Here's how the part is built. I have some questions about the finished solid (model axes, mm). Face numbers are marked on the shaded views. A direction names the side the tool comes from. Coordinates: 2 decimals unless noted, no trailing zeros. Loops run counter-clockwise (first coordinate to the right, second up) from the corner with the lowest first, then second, coordinate; pieces in that order, holes last. Notation, with made-up numbers: (-19, 16) -> (33, 16) arc R22 ccw to (33, 30) -> close; hole circle Ø10 at (-27.75, -40). An arc over 180 degrees is marked (long way). Answer as a JSON object with one key per item and string values. Group by question number.
1) Which directions (+Z, -Z, +X, -X, +Y, -Y) give clear straight access to the entire face, cutting with the end or side of a thin tool? Please do the marked faces 5, 6, 7, 8 and 9.
2) If we mould it in two halves opening along X, with no side actions, what happens to the marked faces 1, 2, 3 and 4? For each: +X half, -X half, draft (parallel to the pull), parting line (faces both ways), or undercut.
3) I'm going to push flat-ended pins straight in: pin 1 (13.5 mm diameter, centred on x = 23, z = 14.5, fed in from -Y); pin 2 (3.5 mm diameter, centred on x = 9, y = -43, fed in from +Z); pin 3 (10 mm diameter, centred on x = 0.5, y = -2, fed in from -Z). Where does each tip first touch, or does it pass through?
4) I want a section at B-B (x = 7.5). Write out the boundary of the cut face in (y, z).
5) I want a section at D-D (y = -34). Write out the boundary of the cut face in (x, z), then the cut area to 3 significant figures.
6) I need wall thicknesses on probe 1 along Y at (x, z) = (-11.5, 25.5); probe 2 along Z at (x, y) = (9, 3). Which ranges of each line are inside material? Lowest first, please. Write a range as [from, to].
7) I want a section at C-C (z = 6). Write out the boundary of the cut face in (x, y), then the cut area to 3 significant figures.
8) I want a section at A-A (y = 19). Write out the boundary of the cut face in (x, z).
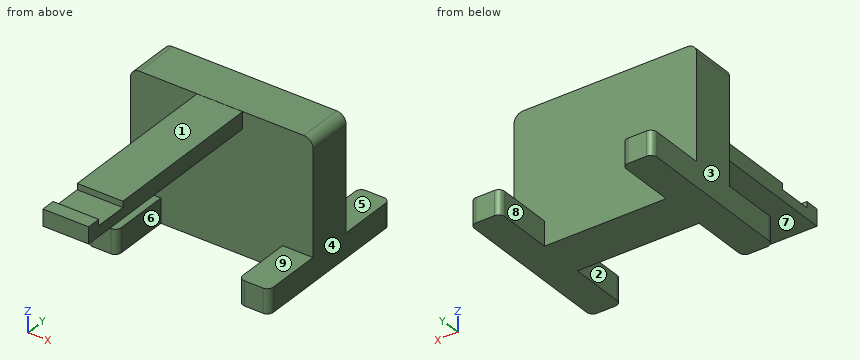
Autodesk Fusion 360 part; units mm, degrees
sketch "Sketch1" plane through (0, 0, 0) normal (0, 0, 1) x (1, 0, 0)
  line L0 (-20, 40) -> (-19.9999, 40)
  line L1 (-19.9999, 10) -> (-20, 10)
  line L2 (-20, 40) -> (40, 40)
  line L3 (40, 40) -> (40, 25)
  line L4 (40, 25) -> (-20, 25)
  line L5 (-20, 25) -> (-20, 40)
  line L6 (20, 40) -> (40, 40)
  dimension "d12" = 60
extrude "Extrude6" add sketch "Sketch1" along normal blind 40
sketch "Sketch5" plane through (0, 25, 0) normal (0, -1, 0) x (1, 0, 0)
  line L0 (-20, 0) -> (40, 0)
  line L1 (40, 0) -> (40, 40)
  line L2 (40, 40) -> (-20, 40)
  line L3 (-20, 40) -> (-20, 0)
  line L4 (1.8726, 40) -> (16.8726, 40)
  line L5 (16.8726, 40) -> (16.8726, 45.446)
  line L6 (16.8726, 45.446) -> (1.8726, 45.446)
  line L7 (1.8726, 45.446) -> (1.8726, 40)
  point P0 (10, 40)
  dimension "d29" = 15
extrude "Extrude7" add sketch "Sketch5" along normal blind 70 contours L2 L4 L5 L6 L7
sketch "Sketch6" plane through (0, 0, 40) normal (0, 0, -1) x (-1, 0, 0)
  line L0 (20, 40) -> (20, 25)
  line L1 (20, 25) -> (-1.8726, 25)
  line L2 (-40, 25) -> (-40, 40)
  line L3 (-40, 40) -> (20, 40)
  line L4 (-1.8726, 25) -> (-16.8726, 25)
  line L5 (-16.8726, 25) -> (-40, 25)
extrude "Extrude8" add sketch "Sketch6" against normal blind 5.5
sketch "Sketch7" plane through (0, 25, 0) normal (0, -1, 0) x (1, 0, 0)
  line L0 (-20, 45.5) -> (-20, 0)
  line L1 (-20, 0) -> (40, 0)
  line L2 (40, 0) -> (40, 45.5)
  line L3 (-20, 8) -> (-10, 8)
  line L4 (-10, 8) -> (-10, 0)
  line L5 (-10, 0) -> (-20, 0)
  line L6 (-20, 0) -> (-20, 8)
  line L7 (30, 8) -> (40, 8)
  line L8 (40, 8) -> (40, 0)
  line L9 (40, 0) -> (30, 0)
  line L10 (30, 0) -> (30, 8)
  line L11 (16.8726, 45.446) -> (16.8726, 40)
  line L12 (1.8726, 40) -> (1.8726, 45.446)
  line L13 (40, 45.5) -> (-20, 45.5)
  line L14 (16.8726, 40) -> (1.8726, 40)
  line L15 (1.8726, 45.446) -> (16.8726, 45.446)
  dimension "d25" = 10
  dimension "d26" = 8
  dimension "d27" = 10
  dimension "d28" = 8
extrude "Extrude9" add sketch "Sketch7" along normal blind 20 contours L0 L1 L3 L4 L5 L6 | L1 L2 L7 L8 L9 L10
sketch "Sketch8" plane through (0, 40, 0) normal (0, 1, 0) x (-1, 0, 0)
  line L0 (-40, 0) -> (20, 0)
  line L1 (20, 0) -> (20, 45.5)
  line L2 (-40, 45.5) -> (-40, 0)
  line L3 (-40, 8) -> (-30, 8)
  line L4 (-30, 8) -> (-30, 0)
  line L5 (-30, 0) -> (-40, 0)
  line L6 (-40, 0) -> (-40, 8)
  line L7 (10, 8) -> (20, 8)
  line L8 (20, 8) -> (20, 0)
  line L9 (20, 0) -> (10, 0)
  line L10 (10, 0) -> (10, 8)
  line L11 (20, 45.5) -> (-40, 45.5)
  dimension "d34" = 10
  dimension "d35" = 8
  dimension "d36" = 8
  dimension "d37" = 10
extrude "Extrude10" add sketch "Sketch8" along normal blind 20 contours L0 L2 L3 L4 L5 L6 | L0 L1 L7 L8 L9 L10
sketch "Sketch10" plane through (0, 0, 45.446) normal (0, 0, 1) x (-1, 0, 0)
  line L0 (-1.8726, -25) -> (-1.8726, 45)
  line L1 (-1.8726, 45) -> (-16.8726, 45)
  line L2 (-16.8726, 45) -> (-16.8726, -25)
  line L3 (-16.8726, 40.4277) -> (-1.8726, 40.4277)
  line L4 (-1.8726, 40.4277) -> (-1.8726, 29.4277)
  line L5 (-1.8726, 29.4277) -> (-16.8726, 29.4277)
  line L6 (-16.8726, 29.4277) -> (-16.8726, 40.4277)
  line L7 (-16.8726, -25) -> (-1.8726, -25)
  dimension "d38" = 11
extrude "Extrude12" cut sketch "Sketch10" against normal blind 2 contours L0 L2 L3 L4 L5 L6
fillet "Fillet1" radius 3 2 edges at (40, 32.5, 45.5) (-20, 32.5, 45.5)
fillet "Fillet2" radius 2 8 edges at (40, 5, 4) (30, 5, 4) (40, 60, 4) (-10, 5, 4) (30, 60, 4) (-10, 60, 4) (-20, 60, 4) (-20, 5, 4)
Determined:
{
 "1": {"face 5": "+Z, +X, -X, +Y", "face 6": "+Z, -Z, -Y", "face 7": "-Z, +X, -X, -Y", "face 8": "+Z, -Z, +Y", "face 9": "+Z, +X, -X, -Y"},
 "2": {"face 1": "draft", "face 2": "undercut", "face 3": "-X half", "face 4": "+X half"},
 "3": {"pin 1": "y = 25", "pin 2": "z = 45.45", "pin 3": "z = 40"},
 "4": {"outline": "(-45, 40) -> (25, 40) -> (25, 0) -> (40, 0) -> (40, 45.5) -> (25, 45.5) -> (25, 45.45) -> (-29.43, 45.45) -> (-29.43, 43.45) -> (-40.43, 43.45) -> (-40.43, 45.45) -> (-45, 45.45) -> close"},
 "5": {"outline": "(1.87, 40) -> (16.87, 40) -> (16.87, 43.45) -> (1.87, 43.45) -> close", "area": "51.7 mm^2"},
 "6": {"probe 1": "[25, 40]", "probe 2": "[40, 45.45]"},
 "7": {"outline": "(-20, 7) arc R2 ccw to (-18, 5) -> (-12, 5) arc R2 ccw to (-10, 7) -> (-10, 25) -> (30, 25) -> (30, 7) arc R2 ccw to (32, 5) -> (38, 5) arc R2 ccw to (40, 7) -> (40, 58) arc R2 ccw to (38, 60) -> (32, 60) arc R2 ccw to (30, 58) -> (30, 40) -> (-10, 40) -> (-10, 58) arc R2 ccw to (-12, 60) -> (-18, 60) arc R2 ccw to (-20, 58) -> close", "area": "1,690 mm^2"},
 "8": {"outline": "(-20, 0) -> (-10, 0) -> (-10, 8) -> (-20, 8) -> close; (1.87, 40) -> (16.87, 40) -> (16.87, 45.45) -> (1.87, 45.45) -> close; (30, 0) -> (40, 0) -> (40, 8) -> (30, 8) -> close"}
}
